from build123d import *

# Parameters (mm, degrees)
F0_W         = 14
F0_H         = 30
F0_R         = 3.925
F1_DEPTH     = 15
F3_DEPTH     = 14.001
F4_R         = 1.6
F4_R_2       = 1
F5_DEPTH     = 14.001
F6_R         = 12
F7_T1_DEPTH  = 10
F7_T3_DEPTH  = 11
F7_T5_DEPTH  = 8
F7_S9_W      = 2
F7_S9_H      = 2
F7_T10_DEPTH = 2
F7_S15_W     = 2
F7_S15_H     = 2
F7_T16_DEPTH = 2
F7_T22_DEPTH = 13
F7_T25_ANGLE = 90
F7_T29_DEPTH = 13
F7_T32_ANGLE = 90


# Not quite as in the source:
# - a fillet or chamfer that OpenCascade refuses, or shapes differently, is made with other operations: its cross-section is extruded or revolved along the edge and cut away or added


with BuildPart() as f1:
    # F0 (on Front) → F1 (new body)
    with BuildSketch(Plane.XZ):
        with Locations((0, 5)):
            Rectangle(F0_W, F0_H)
        Circle(F0_R, mode=Mode.SUBTRACT)
    extrude(amount=F1_DEPTH)

    # F2 (on face) → F3 (cut, through all)
    with BuildSketch(Plane.YZ.offset(7)):
        Polygon((-15, -10), (0, -10), (-5, -5), (-15, -5), align=None)
    extrude(amount=-F3_DEPTH, mode=Mode.SUBTRACT)

    # F4 (on face) → F5 (cut, through all)
    with BuildSketch(Plane.YZ.offset(7)):
        with Locations((-1.9, 8)):
            Circle(F4_R)
        with Locations((-7.5, 0)):
            Circle(F4_R_2)
    extrude(amount=-F5_DEPTH, mode=Mode.SUBTRACT)

    # F6
    f6_edges = [f1.edges().sort_by_distance(p)[0] for p in [
        (0, -15, 20),
    ]]
    fillet(f6_edges, radius=F6_R)

    # F7: fillet of radius 2 on 9 edges, made by hand

    # F7_s2 → F7_t1 (cut)
    with BuildSketch(Plane.YZ.offset(-5)):
        with BuildLine():
            ThreePointArc((-15, -3), (-14.4142135624, -4.4142135624), (-13, -5))
            Line((-13, -5), (-15, -5))
            Line((-15, -5), (-15, -3))
        make_face()
    extrude(amount=F7_T1_DEPTH, mode=Mode.SUBTRACT)

    # F7_s4 → F7_t3 (cut)
    with BuildSketch(Plane.XY.offset(-3)):
        with BuildLine():
            ThreePointArc((7, -13), (6.4142135624, -14.4142135624), (5, -15))
            Line((5, -15), (7, -15))
            Line((7, -15), (7, -13))
        make_face()
        with BuildLine():
            ThreePointArc((-7, -13), (-6.4142135624, -14.4142135624), (-5, -15))
            Line((-5, -15), (-7, -15))
            Line((-7, -15), (-7, -13))
        make_face()
    extrude(amount=F7_T3_DEPTH, mode=Mode.SUBTRACT)

    # F7_s6 → F7_t5 (cut)
    with BuildSketch(Plane.XZ.offset(-5)):
        with BuildLine():
            ThreePointArc((5, 20), (6.4142135624, 19.4142135624), (7, 18))
            Line((7, 18), (7, 20))
            Line((7, 20), (5, 20))
        make_face()
        with BuildLine():
            ThreePointArc((-5, 20), (-6.4142135624, 19.4142135624), (-7, 18))
            Line((-7, 18), (-7, 20))
            Line((-7, 20), (-5, 20))
        make_face()
    extrude(amount=F7_T5_DEPTH, mode=Mode.SUBTRACT)


with BuildPart() as f7_tool8:
    # F7_s9 → F7_t10 (new body)
    with BuildSketch(Plane.YZ.offset(5)):
        with Locations((-14, -4)):
            Rectangle(F7_S9_W, F7_S9_H)
    extrude(amount=F7_T10_DEPTH)

    # F7_s11 → F7_t12 (revolve, cut)
    with BuildSketch(Plane(origin=(5, -13, -3), x_dir=(0, 0.7071067812, 0.7071067812), z_dir=(0, 0.7071067812, -0.7071067812))):
        with BuildLine():
            ThreePointArc((0, -2), (2, 0), (0, 2))
            Line((0, 2), (0, -2))
        make_face()
    revolve(axis=Axis((5, -13, -3), (1, 0, 0)), mode=Mode.SUBTRACT)


with BuildPart() as f1_1:
    add(f1.part)

    # F7_t7: cut F7_tool8
    add(f7_tool8.part, mode=Mode.SUBTRACT)


with BuildPart() as f7_tool14:
    # F7_s15 → F7_t16 (new body)
    with BuildSketch(Plane.YZ.offset(-5)):
        with Locations((-14, -4)):
            Rectangle(F7_S15_W, F7_S15_H)
    extrude(amount=-F7_T16_DEPTH)

    # F7_s17 → F7_t18 (revolve, cut)
    with BuildSketch(Plane(origin=(-5, -13, -3), x_dir=(0, 0.7071067812, 0.7071067812), z_dir=(0, -0.7071067812, 0.7071067812))):
        with BuildLine():
            ThreePointArc((0, -2), (2, 0), (0, 2))
            Line((0, 2), (0, -2))
        make_face()
    revolve(axis=Axis((-5, -13, -3), (-1, 0, 0)), mode=Mode.SUBTRACT)


with BuildPart() as f1_2:
    add(f1_1.part)

    # F7_t13: cut F7_tool14
    add(f7_tool14.part, mode=Mode.SUBTRACT)


with BuildPart() as f7_tool20:
    # F7_s21 → F7_t22 (new body)
    with BuildSketch(Plane.XZ):
        with BuildLine():
            ThreePointArc((-7, -3), (-6.4142135624, -4.4142135624), (-5, -5))
            Line((-5, -5), (-7, -5))
            Line((-7, -5), (-7, -3))
        make_face()
    extrude(amount=F7_T22_DEPTH)

    split(bisect_by=Plane(origin=(0, -5, -5), x_dir=(1, 0, 0), z_dir=(0, -0.7071067812, -0.7071067812)), keep=Keep.TOP)


with BuildPart() as f1_3:
    add(f1_2.part)

    # F7_t19: cut F7_tool20
    add(f7_tool20.part, mode=Mode.SUBTRACT)

    # F7_s24 → F7_t25 (revolve, cut)
    with BuildSketch(Plane.XZ.offset(3)):
        with BuildLine():
            ThreePointArc((-5, 20), (-6.4142135624, 19.4142135624), (-7, 18))
            Line((-7, 18), (-7, 20))
            Line((-7, 20), (-5, 20))
        make_face()
    revolve(axis=Axis((-7, -3, 8), (1, 0, 0)), revolution_arc=F7_T25_ANGLE, mode=Mode.SUBTRACT)


with BuildPart() as f7_tool27:
    # F7_s28 → F7_t29 (new body)
    with BuildSketch(Plane.XZ):
        with BuildLine():
            ThreePointArc((7, -3), (6.4142135624, -4.4142135624), (5, -5))
            Line((5, -5), (7, -5))
            Line((7, -5), (7, -3))
        make_face()
    extrude(amount=F7_T29_DEPTH)

    split(bisect_by=Plane(origin=(0, -5, -5), x_dir=(1, 0, 0), z_dir=(0, -0.7071067812, -0.7071067812)), keep=Keep.TOP)


with BuildPart() as f1_4:
    add(f1_3.part)

    # F7_t26: cut F7_tool27
    add(f7_tool27.part, mode=Mode.SUBTRACT)

    # F7_s31 → F7_t32 (revolve, cut)
    with BuildSketch(Plane.XZ.offset(3)):
        with BuildLine():
            ThreePointArc((7, 18), (6.4142135624, 19.4142135624), (5, 20))
            Line((5, 20), (7, 20))
            Line((7, 20), (7, 18))
        make_face()
    revolve(axis=Axis((7, -3, 8), (1, 0, 0)), revolution_arc=F7_T32_ANGLE, mode=Mode.SUBTRACT)


solid = f1_4.part
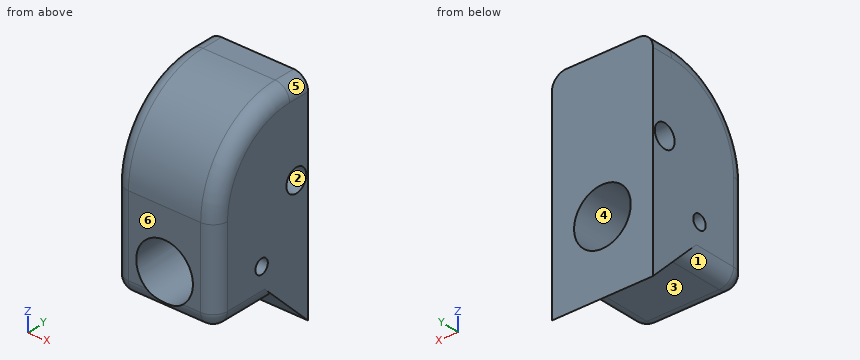
Verification items for the finished model (mm, model axes). Face numbers are marked on the shaded views. A direction names the side the tool comes from. Round coordinates to 2 decimals unless told otherwise and drop trailing zeros. Order: outer loops, then holes, each group sorted by start corner. A loop starts at its lowest first (then second) coordinate and runs counter-clockwise, first axis right, second up.
1. Section check C-C on z = 0. Record the cut outline in (x, y) (3 decimals).
Final values:
outline: (-7, -13) arc R2 ccw to (-5, -15) - (-3.925, -15) - (-3.925, -8.5) - (-7, -8.5) - close; (-7, -6.5) - (-3.925, -6.5) - (-3.925, 0) - (-7, 0) - close; (3.925, -15) - (5, -15) arc R2 ccw to (7, -13) - (7, -8.5) - (3.925, -8.5) - close; (3.925, -6.5) - (7, -6.5) - (7, 0) - (3.925, 0) - close
2. Section check D-D on x = 4.5. Record the cut outline in (y, z).
Final values:
outline: (-15, -3) arc R2 ccw to (-13, -5) - (-5, -5) - (0, -10) - (0, 20) - (-3, 20) arc R12 ccw to (-15, 8) - close; hole circle Ø2 at (-7.5, 0); hole circle Ø3.2 at (-1.9, 8)
3. Go/stop test with flat-tipped pins: P1, Ø4, axis at x = -2, y = -12, coming from the -Z side; P2, Ø6, axis at x = 4, y = -12.5, coming from the +Z side; P3, Ø8, axis at x = -2.5, y = -8.5, coming from the +Z side. Record where each tip stops, or that it passes through.
Final values:
P1: stops at z = -5
P2: stops at z = 18.09
P3: stops at z = 19.91
4. Thickness scan on L1, parallel to Y at x = -5.1, z = 0; L2, parallel to X at y = -10.5, z = 0 (3 decimals); L3, parallel to Z at x = 2.25, y = -1.9. Record the ranges inside material, lowest first.
Final values:
L1: y = -15 to -8.5, -6.5 to 0
L2: x = -7 to -3.925, 3.925 to 7
L3: z = -8.1 to -3.22, 3.22 to 6.4, 9.6 to 20
5. Access from +Z, -Z, +X, -X, +Y, -Y to the whole of each face (thin tool, end or side, straight path). Record for the marked faces 1, 2 and 3.
Final values:
face 1: -Z, -X, -Y
face 2: +X, -X
face 3: -Z, +X, -X, -Y
6. Section check A-A on y = -1.9. Record the cut outline in (x, z) (3 decimals), then the cut area to 3 significant figures.
Final values:
outline: (-7, -8.1) - (7, -8.1) - (7, 6.4) - (-7, 6.4) - close; (-7, 9.6) - (7, 9.6) - (7, 18) arc R2 ccw to (5, 20) - (-5, 20) arc R2 ccw to (-7, 18) - close; hole circle Ø7.85 at (0, 0)
area: 298 mm2
7. Section check B-B on x = -0.5. Record the cut outline in (y, z), then the cut area to 3 significant figures.
Final values:
outline: (-15, 3.89) - (0, 3.89) - (0, 20) - (-3, 20) arc R12 ccw to (-15, 8) - close; (-14.79, -3.89) arc R2 ccw to (-13, -5) - (-5, -5) - (0, -10) - (0, -3.89) - close; hole circle Ø3.2 at (-1.9, 8)
area: 231 mm2
8. Release check for a two-part mould opening along X. For the marked faces 4, 5 and 6 record: +X half, -X half, draft (parallel to the pull), parting line (faces both ways), or undercut.
Final values:
face 4: undercut
face 5: +X half
face 6: draft
